from build123d import *

# Parameters (mm, degrees)
BOX_W           = 17
BOX_H           = 51
BOX_DEPTH       = 12
THICKNESS_T     = 2
POCKET_DEPTH    = 2.001
SKETCH001_W     = 17
SKETCH001_H     = 51
PAD_DEPTH       = 1
POCKET001_DEPTH = 21.001


with BuildPart() as part:
    # Box → Box (new body)
    with BuildSketch(Plane.XY):
        with Locations((8.5, 25.5)):
            Rectangle(BOX_W, BOX_H)
    extrude(amount=BOX_DEPTH)

    # Thickness
    thickness_openings = [part.faces().sort_by_distance(p)[0] for p in [
        (8.5, 25.5, 0),
    ]]
    offset(amount=THICKNESS_T, openings=thickness_openings)

    # Sketch (on Face5 of Thickness) → Pocket (cut, through all)
    with BuildSketch(Plane(origin=(0, 0, 12), x_dir=(1, 0, 0), z_dir=(0, 0, -1))):
        with BuildLine():
            ThreePointArc((11, -5), (8.5, -2.5), (6, -5))
            Line((6, -5), (6, -46))
            ThreePointArc((6, -46), (8.5, -48.5), (11, -46))
            Line((11, -46), (11, -5))
        make_face()
    extrude(amount=-POCKET_DEPTH, mode=Mode.SUBTRACT)

    # Sketch001 (on Face3 of Pocket) → Pad (join)
    with BuildSketch(Plane(origin=(0, 0, 12), x_dir=(1, 0, 0), z_dir=(0, 0, -1))):
        with Locations((8.5, -25.5)):
            Rectangle(SKETCH001_W, SKETCH001_H)
        with BuildLine():
            ThreePointArc((11, -5), (8.5, -2.5), (6, -5))
            Line((6, -5), (6, -46))
            ThreePointArc((6, -46), (8.5, -48.5), (11, -46))
            Line((11, -46), (11, -5))
        make_face(mode=Mode.SUBTRACT)
    extrude(amount=PAD_DEPTH)

    # Sketch002 (on Face17 of Pad) → Pocket001 (cut, through all)
    with BuildSketch(Plane.YZ.offset(19)):
        with BuildLine():
            ThreePointArc((36.076138, 7.358207), (35.076138, 6.358207), (36.076138, 5.358207))
            Line((36.076138, 5.358207), (43.44347, 5.358207))
            ThreePointArc((43.44347, 5.358207), (44.44347, 6.358207), (43.44347, 7.358207))
            Line((43.44347, 7.358207), (36.076138, 7.358207))
        make_face()
        with BuildLine():
            ThreePointArc((5.278592, 7.358207), (4.278592, 6.358207), (5.278592, 5.358207))
            Line((5.278592, 5.358207), (14.177313, 5.358207))
            ThreePointArc((14.177313, 5.358207), (15.177313, 6.358207), (14.177313, 7.358207))
            Line((14.177313, 7.358207), (5.278592, 7.358207))
        make_face()
    extrude(amount=-POCKET001_DEPTH, mode=Mode.SUBTRACT)


solid = part.part
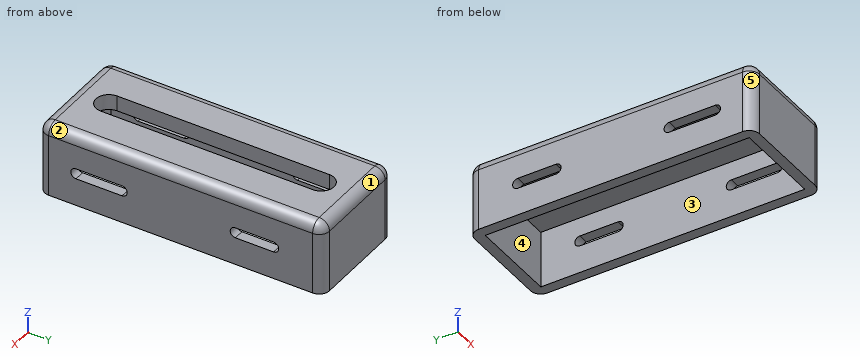
Verification items for the finished model (mm, model axes). Face numbers are marked on the shaded views. A direction names the side the tool comes from. Round coordinates to 2 decimals unless told otherwise and drop trailing zeros. Loops run counter-clockwise (first coordinate to the right, second up) from the corner with the lowest first, then second, coordinate; pieces in that order, holes last. Notation, with made-up numbers: (-20.5, 70) - (10.5, 70) arc R32 ccw to (10.5, 108) - close; hole circle Ø8 at (-33, 65). An arc over 180 degrees is marked (long way). Write item = value, one per line.
Q1. Depth check by flat-ended pin: pin 1 (1 mm diameter, centred on x = 18, y = 41.5, fed in from +Z); pin 2 (0.9 mm diameter, centred on y = 31.5, z = 13, fed in from -X); pin 3 (1.5 mm diameter, centred on x = 13, y = 33, fed in from -Z). Enter the tip coordinate at first touch or a pass-through.
Here are the results:
pin_1 = 13.94
pin_2 = -1.92
pin_3 = 11
Q2. Sectioned sample at C-C on y = 34.5. Record the boundary of the cut face in (x, z), plus the area to 3 significant figures.
Here are the results:
outline = (-2, 0) - (0, 0) - (0, 11) - (6, 11) - (6, 14) - (0, 14) arc R2 ccw to (-2, 12) - close; (11, 11) - (17, 11) - (17, 0) - (19, 0) - (19, 12) arc R2 ccw to (17, 14) - (11, 14) - close
area = 90.3 mm^2
Q3. Sectioned sample at B-B on x = 7. Record the boundary of the cut face in (y, z).
Here are the results:
outline = (-2, 0) - (0, 0) - (0, 11) - (3, 11) - (3, 14) - (0, 14) arc R2 ccw to (-2, 12) - close; (48, 11) - (51, 11) - (51, 0) - (53, 0) - (53, 12) arc R2 ccw to (51, 14) - (48, 14) - close
Q4. Sectioned sample at D-D on z = 4. Record the boundary of the cut face in (x, y), plus the area to 3 significant figures.
Here are the results:
outline = (-2, 0) arc R2 ccw to (0, -2) - (17, -2) arc R2 ccw to (19, 0) - (19, 51) arc R2 ccw to (17, 53) - (0, 53) arc R2 ccw to (-2, 51) - close; hole (0, 0) - (17, 0) - (17, 51) - (0, 51) - close
area = 285 mm^2
Q5. Material ranges on L1, parallel to X at y = 22.5, z = 3.5; L2, parallel to Y at x = 11, z = 9.25; L3, parallel to X at y = 43, z = 12, recorded low to high.
Here are the results:
L1 = -2 to 0, 17 to 19
L2 = -2 to 0, 51 to 53
L3 = -2 to 6, 11 to 19
Q6. Sectioned sample at A-A on y = 9. Record the boundary of the cut face in (x, z).
Here are the results:
outline = (-2, 0) - (0, 0) - (0, 5.36) - (-2, 5.36) - close; (-2, 7.36) - (0, 7.36) - (0, 11) - (6, 11) - (6, 14) - (0, 14) arc R2 ccw to (-2, 12) - close; (11, 11) - (17, 11) - (17, 7.36) - (19, 7.36) - (19, 12) arc R2 ccw to (17, 14) - (11, 14) - close; (17, 0) - (19, 0) - (19, 5.36) - (17, 5.36) - close
Q7. Tool access check on the marked faces 4 and 5. Record the directions out of +Z, -Z, +X, -X, +Y, -Y that give a thin tool (end or side, any length) a straight path to the whole face; none if there is none.
Here are the results:
face_4 = -Z
face_5 = +Z, -Z, -X, -Y
Q8. Mould release check, pull along Y, two halves, no side actions. Record for the marked faces 1, 2 and 3: +Y half, -Y half, draft (parallel to the pull), parting line (faces both ways), or undercut.
Here are the results:
face_1 = +Y half
face_2 = draft
face_3 = undercut
